```python
from build123d import *

# Parameters (mm, degrees)
SKIZZE1_W                        = 35
SKIZZE1_H                        = 75
AUFSATZ_LINEAR_AUSTRAGEN1_DEPTH  = 1.5
SKIZZE3_W                        = 15.25
SKIZZE3_H                        = 5
SKIZZE3_W_2                      = 4.875
SCHNITT_LINEAR_AUSTRAGEN12_DEPTH = 20
SKIZZE4_RX                       = 23.75
SKIZZE4_RY                       = 12
SKIZZE4_RX_2                     = 22.75
SKIZZE4_RY_2                     = 11
SCHNITT_LINEAR_AUSTRAGEN13_DEPTH = 20
SKIZZE6_W                        = 1
SKIZZE6_H                        = 52.800334248
AUFSATZ_LINEAR_AUSTRAGEN4_DEPTH  = 1.5


with BuildPart() as part:
    # Skizze1 → Aufsatz-Linear austragen1 (new body)
    with BuildSketch(Plane.XY):
        with Locations((17.5, 37.5)):
            Rectangle(SKIZZE1_W, SKIZZE1_H)
    extrude(amount=AUFSATZ_LINEAR_AUSTRAGEN1_DEPTH)

    # Skizze3 → Schnitt-Linear austragen12 (cut)
    with BuildSketch(Plane.XY.offset(1.5)):
        with Locations((17.5, 2.5)):
            Rectangle(SKIZZE3_W, SKIZZE3_H)
        with Locations((32.5625, 2.5)):
            Rectangle(SKIZZE3_W_2, SKIZZE3_H)
        with Locations((2.4375, 2.5)):
            Rectangle(SKIZZE3_W_2, SKIZZE3_H)
    extrude(amount=-SCHNITT_LINEAR_AUSTRAGEN12_DEPTH, mode=Mode.SUBTRACT)

    # Skizze4 → Schnitt-Linear austragen13 (cut)
    with BuildSketch(Plane.XY.offset(1.5)):
        with Locations(Location((17.5, 40.75), (0, 0, 90))):
            Ellipse(SKIZZE4_RX, SKIZZE4_RY)
        with Locations(Location((17.5, 40.75), (0, 0, 90))):
            Ellipse(SKIZZE4_RX_2, SKIZZE4_RY_2, mode=Mode.SUBTRACT)
    extrude(amount=-SCHNITT_LINEAR_AUSTRAGEN13_DEPTH, mode=Mode.SUBTRACT)


with BuildPart() as schnitt_linear_austragen13_piece_1:
    # of the separate pieces the step leaves, piece 1, a body of its own (schnitt_linear_austragen13_pieces)
    add(part.part.solids().sort_by_distance((4.875, 0, 0))[0])



with BuildPart() as schnitt_linear_austragen13_piece_2:
    # of the separate pieces the step leaves, piece 2, a body of its own (schnitt_linear_austragen13_pieces)
    add(part.part.solids().sort_by_distance((17.5, 63.5, 0))[0])


with BuildPart() as schnitt_linear_austragen13_piece_1_1:
    add(schnitt_linear_austragen13_piece_1.part)

    add(schnitt_linear_austragen13_piece_2.part)  # Aufsatz-Linear austragen4 merges Schnitt-Linear austragen13 piece 2
    # Skizze6 → Aufsatz-Linear austragen4 (add)
    with BuildSketch(Plane.XY.offset(1.5)):
        with Locations((17.5, 39.413172243)):
            Rectangle(SKIZZE6_W, SKIZZE6_H)
    extrude(amount=-AUFSATZ_LINEAR_AUSTRAGEN4_DEPTH)


solid = schnitt_linear_austragen13_piece_1_1.part
```
Model file for the job. Use its own axes, mm. A direction names the side the tool comes from. Coordinates: 2 decimals unless noted, no trailing zeros. Write each loop counter-clockwise with the first axis right and the second up, starting at its lowest first coordinate (ties: lowest second). Pieces come first, ordered by that corner, then holes. Notation, with made-up numbers: (9.25, 20) - (68.25, 20) arc R24 ccw to (68.25, 32) - close; hole circle Ø1 at (24, 28.5). An arc over 180 degrees is marked (long way). One line per item, written item: value. Start each with the question number.
1. Flat gauge pin, fed straight in: pin 1 (0.8 mm diameter, centred on x = 31.5, z = 0.5, fed in from -Y). Where does the tip first touch, or does it go through?
2. Probe line 1 (X direction, y = 28.5, z = 1.4); line 2 (X direction, y = 25.5, z = 0.35); line 3 (Y direction, x = 19, z = 0.5). List the from-to ranges inside material, lowest first. Write a range as from..to.
3. Tool access for faces 1 (the flat face through (2, 5, 1)), 2 (the flat face through (30.125, 2, 1)), 3 (the flat face through (25.125, 2, 1)): list every direction of +Z, -Z, +X, -X, +Y, -Y with a clear straight run to the whole face (end or side of a thin tool).
4. Slice it at A-A (x = 27.5). Count the separate pieces of the cut face and the enclosed holes in it, plus the area to 3 significant figures.
5. Slice it at D-D (x = 4). Write the cut outline in (y, z), plus the area to 3 significant figures.
6. Mould opens along X. For faces 4 (the flat face through (17, 38, 1.5)), 5 (the flat face through (4.875, 2, 1)), 6 (the flat face through (9.875, 2, 1)) say: released by +X, released by -X, zero draft, split by the parting line, or undercut.
Answers below:
1. pin 1: stops at y = 5
2. line 1: x = 0..7.22, 8.23..26.77, 27.78..35
2. line 2: x = 0..8.3, 9.34..25.66, 26.7..35
2. line 3: y = 5..17.19, 18.21..63.29, 64.31..75
3. face 1: +Z, -Z, -X, -Y
3. face 2: +Z, -Z, +X, -Y
3. face 3: +Z, -Z, -Y
4. separate pieces: 3
4. enclosed holes: 0
4. area: 102 mm^2
5. outline: (5, 0) - (75, 0) - (75, 1.5) - (5, 1.5) - close
5. area: 105 mm^2
6. face 4: zero draft
6. face 5: released by -X
6. face 6: undercut
